```python
from build123d import *

# Parameters (mm, degrees)
SKETCH1_W           = 58
SKETCH1_H           = 10
SKETCH1_R           = 2
BOSS_EXTRUDE1_DEPTH = 45
SKETCH3_W           = 58
SKETCH3_H           = 10
CUT_EXTRUDE3_DEPTH  = 10
SKETCH4_R           = 5
CUT_EXTRUDE4_DEPTH  = 10


with BuildPart() as part:
    # Sketch1 → Boss-Extrude1 (new body)
    with BuildSketch(Plane.XY):
        with Locations((29, -5)):
            Rectangle(SKETCH1_W, SKETCH1_H)
        with Locations(Location((14, -5, 0), (0, 0, 180))):
            Circle(SKETCH1_R, mode=Mode.SUBTRACT)
        with Locations(Location((44, -5, 0), (0, 0, 180))):
            Circle(SKETCH1_R, mode=Mode.SUBTRACT)
    extrude(amount=BOSS_EXTRUDE1_DEPTH)

    # Sketch3 → Cut-Extrude3 (cut)
    with BuildSketch(Plane(origin=(0, 0, 0), x_dir=(-1, 0, 0), z_dir=(0, 0, -1))):
        with Locations((-29, -5)):
            Rectangle(SKETCH3_W, SKETCH3_H)
    extrude(amount=-CUT_EXTRUDE3_DEPTH, mode=Mode.SUBTRACT)

    # Sketch4 → Cut-Extrude4 (cut)
    with BuildSketch(Plane(origin=(0, 0, 0), x_dir=(1, 0, 0), z_dir=(0, 1, 0))):
        with Locations(Location((29, -21.5, 0), (0, 0, 270))):
            Circle(SKETCH4_R)
    extrude(amount=-CUT_EXTRUDE4_DEPTH, mode=Mode.SUBTRACT)


solid = part.part
```
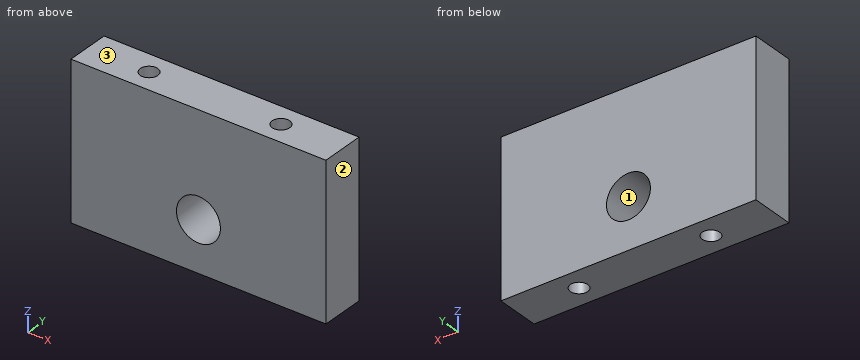
Geometry: final body of the model. Coordinates: model frame, mm. Face numbers are marked on the shaded views. Coordinates: 2 decimals unless noted, no trailing zeros. Loops run counter-clockwise (first coordinate to the right, second up) from the corner with the lowest first, then second, coordinate; pieces in that order, holes last. Notation, with made-up numbers: M 50,39.25 L 56,39.25 A25 cw 56,67.25 Z; hole C 47.25,-34 d2. An arc over 180 degrees is marked long. Put each result on its own line as item: value.
(1) Draft query along X for the marked faces 1, 2 and 3. Return one class per face: pulls with the +X half, pulls with the -X half, needs draft (parallel to the pull), parting line crosses it, or undercut.
Answer sheet:
face 1: undercut
face 2: pulls with the +X half
face 3: needs draft
(2) First-contact query: pin 1 (5 mm diameter, centred on x = 24, z = 29, fed in from +Y); pin 2 (2.5 mm diameter, centred on x = 14, y = -5, fed in from -Z). Flat tips, straight axial feed; report the tip coordinate or a pass-through.
Answer sheet:
pin 1: stops at y = 0
pin 2: passes through
(3) Cut plane A-A on y = -5. Return the cut outline in (x, z).
Answer sheet:
outline: M 0,10 L 12,10 L 12,45 L 0,45 Z; M 16,10 L 42,10 L 42,45 L 16,45 Z; M 46,10 L 58,10 L 58,45 L 46,45 Z; hole C 29,21.5 d10
(4) Cut plane B-B on z = 21.5. Return the cut outline in (x, y), then the cut area to 3 significant figures.
Answer sheet:
outline: M 0,-10 L 24,-10 L 24,0 L 0,0 Z; M 34,-10 L 58,-10 L 58,0 L 34,0 Z; hole C 14,-5 d4; hole C 44,-5 d4
area: 455 mm^2
(5) Material intervals for probe 1 along X at (y, z) = (-5, 36); probe 2 along X at (y, z) = (-6.5, 17.5); probe 3 along Y at (x, z) = (44, 35.5), sorted ascending.
Answer sheet:
probe 1: x = 0 to 12, 16 to 42, 46 to 58
probe 2: x = 0 to 12.68, 15.32 to 26, 32 to 42.68, 45.32 to 58
probe 3: y = -10 to -7, -3 to 0
(6) Cut plane D-D on y = -1.75. Return the cut outline in (x, z).
Answer sheet:
outline: M 0,10 L 58,10 L 58,45 L 0,45 Z; hole C 29,21.5 d10
(7) Cut plane C-C on x = 44. Return the cut outline in (y, z).
Answer sheet:
outline: M -10,10 L -7,10 L -7,45 L -10,45 Z; M -3,10 L 0,10 L 0,45 L -3,45 Z
